Source: CAD feature listing. Evaluate the final solid. Frame: model axes, mm. Face numbers are marked on the shaded views. A direction names the side the tool comes from. Give positions to 0.01 mm unless a question says otherwise; leave off trailing zeros. Order: outer loops, then holes, each group sorted by start corner. A loop starts at its lowest first (then second) coordinate and runs counter-clockwise, first axis right, second up. Notation, with made-up numbers: (81.25, 12) - (135.25, 12) arc R27 ccw to (135.25, 44) - close; hole circle Ø3 at (11, -38). An arc over 180 degrees is marked (long way). Use CSV: the item, a comma, the result in double quotes.
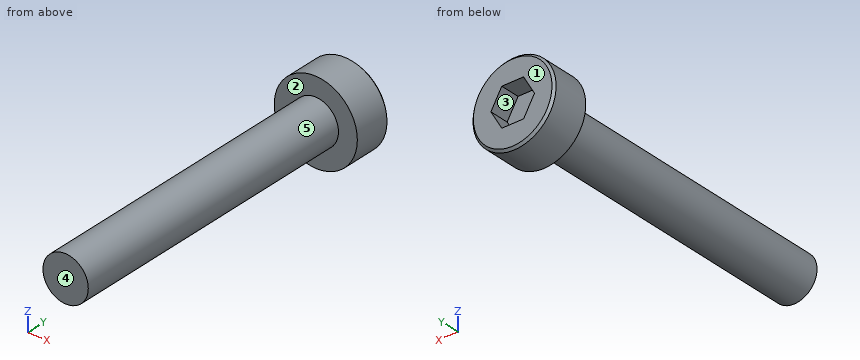
Solid Edge part; units mm, degrees
sketch "Sketch1" plane through (0, 0, 0) normal (0, -1, 0) x (1, 0, 0)
  circle A0 centre (0, 0) radius 1.5
extrude "Protrusion1" add sketch "Sketch1" against normal blind 20
sketch "Sketch2" plane through (0, 20, 0) normal (0, 1, 0) x (1, 0, 0)
  circle A0 centre (0, 0) radius 2.75
extrude "ExtrudedProtrusion_2" add sketch "Sketch2" along normal blind 2.52
sketch "Sketch3" plane through (0, 22.52, 0) normal (0, 1, 0) x (-1, 0, 0)
  line L0 (0.7217, 1.25) -> (-0.7217, 1.25)
  line L1 (-0.7217, 1.25) -> (-1.4434, 0)
  line L2 (-1.4434, 0) -> (-0.7217, -1.25)
  line L3 (-0.7217, -1.25) -> (0.7217, -1.25)
  line L4 (0.7217, -1.25) -> (1.4434, 0)
  line L5 (1.4434, 0) -> (0.7217, 1.25)
extrude "Cutout1" cut sketch "Sketch3" against normal blind 1.3
chamfer "Chamfer_1" distance 0.15 angle 45 1 edges at (-2.75, 22.52, 0)
properties material "Nylon, general purpose"
Item 1: Mould query, pull axis Z, two halves, no side actions, for the marked faces 3, 4 and 5. Classes: released by +Z, released by -Z, zero draft, split by the parting line, or undercut.
Filled in:
face 3,"undercut"
face 4,"zero draft"
face 5,"split by the parting line"
Item 2: Set-up query: the marked faces 1 and 2. Return all of +Z, -Z, +X, -X, +Y, -Y with unobstructed straight access to the full face (end or side cutting, diameter ignored); none if empty.
Filled in:
face 1,"+Z, -Z, +X, -X, +Y"
face 2,"-Y"
Item 3: First-contact query: pin 1 (1 mm diameter, centred on x = -0.5, y = 14.5, fed in from -Z); pin 2 (2 mm diameter, centred on y = 5.5, z = 0.5, fed in from +X). Flat tips, straight axial feed; report the tip coordinate or a pass-through.
Filled in:
pin 1,"stops at z = -1.5"
pin 2,"stops at x = 1.5"
Item 4: Section A-A on x = 0. Return the cut outline in (y, z).
Filled in:
outline,"(0, -1.5) - (20, -1.5) - (20, -2.75) - (22.37, -2.75) - (22.52, -2.6) - (22.52, -1.25) - (21.22, -1.25) - (21.22, 1.25) - (22.52, 1.25) - (22.52, 2.6) - (22.37, 2.75) - (20, 2.75) - (20, 1.5) - (0, 1.5) - close"
Item 5: Material intervals for line 1 (Y direction, x = -2.15, z = 0.5); line 2 (Y direction, x = -0.15, z = 1.1); line 3 (X direction, y = 8.25, z = -0.1), sorted ascending. Write a range as from..to.
Filled in:
line 1,"y = 20..22.52"
line 2,"y = 0..21.22"
line 3,"x = -1.5..1.5"
Item 6: Section B-B on y = 2. Return the cut outline in (x, z).
Filled in:
outline,"circle Ø3 at (0, 0)"
